from build123d import *

# Parameters (mm, degrees)
SKETCH1_R           = 5
BOSS_EXTRUDE1_DEPTH = 191.48
SKETCH2_R           = 6
BOSS_EXTRUDE2_DEPTH = 2
SKETCH3_R           = 5
CUT_EXTRUDE1_DEPTH  = 35.74
SKETCH4_R           = 5
CUT_EXTRUDE2_DEPTH  = 35.74


with BuildPart() as part:
    # Sketch1 → Boss-Extrude1 (new body)
    with BuildSketch(Plane.XY):
        Circle(SKETCH1_R)
    extrude(amount=BOSS_EXTRUDE1_DEPTH)

    # Sketch2 → Boss-Extrude2 (add)
    with BuildSketch(Plane.XY.offset(105.74)):
        Circle(SKETCH2_R)
    boss_extrude2 = extrude(amount=BOSS_EXTRUDE2_DEPTH)

    # Mirror1: Boss-Extrude2 across plane
    add(boss_extrude2.mirror(Plane.XY.offset(95.74)))

    # Sketch3 → Cut-Extrude1 (cut)
    with BuildSketch(Plane.XY.offset(191.48)):
        Circle(SKETCH3_R)
    extrude(amount=-CUT_EXTRUDE1_DEPTH, mode=Mode.SUBTRACT)

    # Sketch4 → Cut-Extrude2 (cut)
    with BuildSketch(Plane(origin=(0, 0, 0), x_dir=(-1, 0, 0), z_dir=(0, 0, -1))):
        Circle(SKETCH4_R)
    extrude(amount=-CUT_EXTRUDE2_DEPTH, mode=Mode.SUBTRACT)


solid = part.part
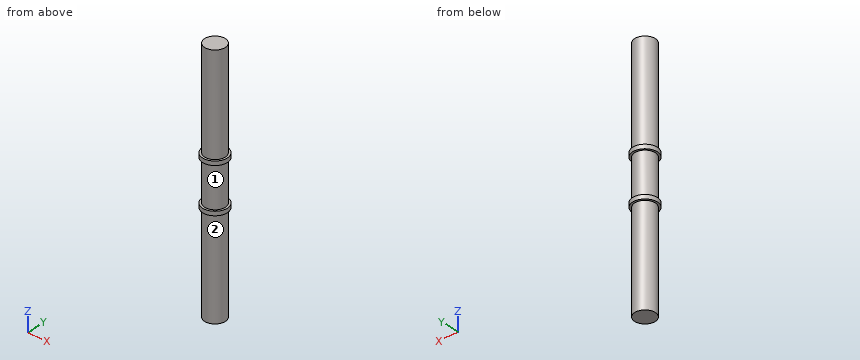
The model under review builds one solid part; all positions refer to its coordinate system, in mm. Face numbers are marked on the shaded views. Coordinates: 2 decimals unless noted, no trailing zeros. Loops run counter-clockwise (first coordinate to the right, second up) from the corner with the lowest first, then second, coordinate; pieces in that order, holes last. Notation, with made-up numbers: M -21.5,-29.5 L 8.5,-29.5 A33 cw 8.5,6.5 Z; hole C 10.5,48 d4. An arc over 180 degrees is marked long. Put each result on its own line as item: value. Start each with the question number.
Q1. Clearance check with flat-ended pins moving along their axes: pin 1 (3 mm diameter, centred on x = 0, z = 112.5, fed in from +Y); pin 2 (3 mm diameter, centred on y = -4.5, z = 82.5, fed in from -X); pin 3 (1.5 mm diameter, centred on y = 3.5, z = 82, fed in from -X). State where each tip first meets the part, or that it passes through.
Q2. Wall thickness on line 1 (Z direction, x = -3, y = -4.5); line 2 (X direction, y = 0, z = 92); line 3 (Y direction, x = 2.75, z = 112): over which ranges is each line inside the solid? List them lowest first.
Q3. The part is to be moulded in two halves that separate along Z. For the marked faces 1 and 2, say which applies: +Z half, -Z half, draft (parallel to the pull), parting line (faces both ways), or undercut.
Q4. Add section C-C (z = 46.5). Write out the cut boundary in (x, y).
Q5. Add section A-A (y = 0). Write out the cut boundary in (x, z).
Answers:
1. pin 1: stops at y = 5
1. pin 2: stops at x = -4.76
1. pin 3: stops at x = -4.18
2. line 1: z = 83.74 to 85.74, 105.74 to 107.74
2. line 2: x = -5 to 5
2. line 3: y = -4.18 to 4.18
3. face 1: undercut
3. face 2: draft
4. outline: C 0,0 d10
5. outline: M -6,83.74 L -5,83.74 L -5,35.74 L 5,35.74 L 5,83.74 L 6,83.74 L 6,85.74 L 5,85.74 L 5,105.74 L 6,105.74 L 6,107.74 L 5,107.74 L 5,155.74 L -5,155.74 L -5,107.74 L -6,107.74 L -6,105.74 L -5,105.74 L -5,85.74 L -6,85.74 Z
